from build123d import *

# Parameters (mm, degrees)
SKETCH1_W           = 28.575
SKETCH1_H           = 50.8
BOSS_EXTRUDE1_DEPTH = 1.5875
BOSS_EXTRUDE2_DEPTH = 14.2875
SKETCH1_4_W         = 25.4
SKETCH1_4_H         = 25.4
SKETCH1_4_W_2       = 22.225
SKETCH1_4_H_2       = 22.225
BOSS_EXTRUDE3_DEPTH = 1016
BOSS_EXTRUDE4_DEPTH = 12.7
LPATTERN1_COUNT     = 2
LPATTERN1_PITCH     = 25.4


with BuildPart() as part:
    # Sketch1 → Boss-Extrude1 (new body)
    with BuildSketch(Plane(origin=(0, 0, 0), x_dir=(0, 0, -1), z_dir=(1, 0, 0))):
        Rectangle(SKETCH1_W, SKETCH1_H)
    extrude(amount=-BOSS_EXTRUDE1_DEPTH)

    # Sketch1<3> → Boss-Extrude2 (add)
    with BuildSketch(Plane(origin=(0, 0, 0), x_dir=(0, 0, -1), z_dir=(1, 0, 0))):
        Polygon((-12.7, 12.7), (-12.7, 25.4), (-14.2875, 25.4), (-14.2875, -25.4), (-12.7, -25.4), (-12.7, -12.7), align=None)
        Polygon((14.2875, 25.4), (12.7, 25.4), (12.7, 12.7), (12.7, -12.7), (12.7, -25.4), (14.2875, -25.4), align=None)
    extrude(amount=-BOSS_EXTRUDE2_DEPTH)

    # Sketch1<4> → Boss-Extrude3 (add)
    with BuildSketch(Plane(origin=(0, 0, 0), x_dir=(0, 0, -1), z_dir=(1, 0, 0))):
        Rectangle(SKETCH1_4_W, SKETCH1_4_H)
        Rectangle(SKETCH1_4_W_2, SKETCH1_4_H_2, mode=Mode.SUBTRACT)
    extrude(amount=BOSS_EXTRUDE3_DEPTH)

    # 3DSketch1 → Boss-Extrude4 (add)
    with BuildSketch(Plane(origin=(-1.5875, 12.7, -6.35), x_dir=(0, 1, 0), z_dir=(0, 0, 1))):
        Polygon((0, 0), (0, 3.175), (6.35, 0), align=None)
    boss_extrude4 = extrude(amount=BOSS_EXTRUDE4_DEPTH)

    # LPattern1: Boss-Extrude4 ×2
    with Locations(*[(0, -i * LPATTERN1_PITCH, 0) for i in range(1, LPATTERN1_COUNT)]):
        add(boss_extrude4)


solid = part.part
Verification items for the finished model (mm, model axes). A direction names the side the tool comes from. Round coordinates to 2 decimals unless told otherwise and drop trailing zeros. Order: outer loops, then holes, each group sorted by start corner. A loop starts at its lowest first (then second) coordinate and runs counter-clockwise, first axis right, second up. Notation, with made-up numbers: (-2, -12) -> (37, -12) arc R9 ccw to (37, 4) -> close; hole circle Ø1 at (-15.75, 24). An arc over 180 degrees is marked (long way). Put each result on its own line as item: value.
1) Material ranges on line 1 (Y direction, x = 165.5, z = 1); line 2 (X direction, y = 2, z = -13), recorded low to high.
Final values:
line 1: y = -12.7 to -11.11, 11.11 to 12.7
line 2: x = -14.29 to 0
2) Section check B-B (z = 0.5). Record the cut outline in (x, y), then the cut area to 3 significant figures.
Final values:
outline: (-4.76, -12.7) -> (-1.59, -12.7) -> (-1.59, -25.4) -> (0, -25.4) -> (0, -12.7) -> (1016, -12.7) -> (1016, -11.11) -> (0, -11.11) -> (0, 11.11) -> (1016, 11.11) -> (1016, 12.7) -> (0, 12.7) -> (0, 25.4) -> (-1.59, 25.4) -> (-1.59, 19.05) -> (-4.76, 12.7) -> (-1.59, 12.7) -> (-1.59, -6.35) -> close
area: 3,330 mm^2
3) Mould release check, pull along Z, two halves, no side actions. Record for faces 4 (the flat face through (501, 12.7, 0)), 5 (the flat face through (501, 0, -11.112)), 6 (the flat face through (501, 0, 12.7)): +Z half, -Z half, draft (parallel to the pull), parting line (faces both ways), or undercut.
Final values:
face 4: draft
face 5: undercut
face 6: +Z half
4) Depth check by flat-ended pin: pin 1 (11 mm diameter, centred on x = 537.5, z = 4, fed in from +Y); pin 2 (3 mm diameter, centred on x = 483.5, y = -4.5, fed in from +Z); pin 3 (1.5 mm diameter, centred on x = 850, z = 1, fed in from -Y); pin 4 (5 mm diameter, centred on x = 637, y = -15.5, fed in from +Z). Enter the tip coordinate at first touch or a pass-through.
Final values:
pin 1: stops at y = 12.7
pin 2: stops at z = 12.7
pin 3: stops at y = -12.7
pin 4: passes through
5) Set-up check for faces 1 (the flat face through (501, -12.7, 0)), 2 (the flat face through (501, 11.112, 0)), 3 (the flat face through (501, 0, -12.7)): record each of +Z, -Z, +X, -X, +Y, -Y from which the full face is reachable in a straight line by a thin tool's end or side.
Final values:
face 1: +Z, -Z, +X, -Y
face 2: +X
face 3: -Z, +X, +Y, -Y
6) Section check A-A (x = 950). Record the cut outline in (y, z), then the cut area to 3 significant figures.
Final values:
outline: (-12.7, -12.7) -> (12.7, -12.7) -> (12.7, 12.7) -> (-12.7, 12.7) -> close; hole (-11.11, -11.11) -> (11.11, -11.11) -> (11.11, 11.11) -> (-11.11, 11.11) -> close
area: 151 mm^2
